Work out the finished part from the listing and answer in its coordinate system (mm). A direction names the side the tool comes from. Give positions to 0.01 mm unless a question says otherwise; leave off trailing zeros. Loops run counter-clockwise (first coordinate to the right, second up) from the corner with the lowest first, then second, coordinate; pieces in that order, holes last. Notation, with made-up numbers: (-4.75, -34) - (15.25, -34) arc R33 cw to (15.25, 5) - close; hole circle Ø10 at (71, -4.75). An arc over 180 degrees is marked (long way). Use CSV: the item, a comma, the result in double quotes.
from build123d import *

# Parameters (mm, degrees)
SKETCH1_R           = 4.25
SKETCH1_R_2         = 1.05
BOSS_EXTRUDE1_DEPTH = 23
BOSS_EXTRUDE3_DEPTH = 2
SKETCH4_W           = 21
SKETCH4_H           = 41
CUT_EXTRUDE1_DEPTH  = 50.288548817
BOSS_EXTRUDE4_START = 42
BOSS_EXTRUDE4_DEPTH = 42
CUT_EXTRUDE4_REACH  = 70.367


with BuildPart() as part:
    # Sketch1 → Boss-Extrude1 (new, symmetric)
    with BuildSketch(Plane.XY):
        with BuildLine():
            Line((-0.798015115, 9.968107738), (11.201984885, 9.968107738))
            ThreePointArc((11.201984885, 9.968107738), (19.90012903, 28.53283063), (7.687881875, 45))
            Line((7.687881875, 45), (3.464101615, 45))
            Line((3.464101615, 45), (0, 47))
            Line((0, 47), (10.5, 47))
            ThreePointArc((10.5, 47), (22.975048867, 25.465576737), (8.550692083, 5.18513885))
            ThreePointArc((8.550692083, 5.18513885), (-4.554689659, -8.902516617), (-0.798015115, 9.968107738))
        make_face()
        Circle(SKETCH1_R, mode=Mode.SUBTRACT)
        with Locations((0, 7)):
            Circle(SKETCH1_R_2, mode=Mode.SUBTRACT)
        with Locations((7, 0)):
            Circle(SKETCH1_R_2, mode=Mode.SUBTRACT)
        with Locations((0, -7)):
            Circle(SKETCH1_R_2, mode=Mode.SUBTRACT)
        with Locations((-7, 0)):
            Circle(SKETCH1_R_2, mode=Mode.SUBTRACT)
    extrude(amount=BOSS_EXTRUDE1_DEPTH, both=True)

    # Sketch3 → Boss-Extrude3 (add)
    with BuildSketch(Plane.XY.offset(23)):
        with BuildLine():
            Line((0, 47), (3.464101615, 45))
            Line((3.464101615, 45), (7.687881875, 45))
            ThreePointArc((7.687881875, 45), (19.90012903, 28.53283063), (11.201984885, 9.968107738))
            Line((11.201984885, 9.968107738), (0, 9.968107738))
            Line((0, 9.968107738), (0, 47))
        make_face()
    boss_extrude3 = extrude(amount=-BOSS_EXTRUDE3_DEPTH)

    # Mirror1: Boss-Extrude3 across plane
    add(boss_extrude3.mirror(Plane.XY))

    # Sketch4 → Cut-Extrude1 (cut, through all)
    with BuildSketch(Plane(origin=(0, 9.968107738, 0), x_dir=(1, 0, 0), z_dir=(0, 1, 0))):
        Rectangle(SKETCH4_W, SKETCH4_H)
    extrude(amount=-CUT_EXTRUDE1_DEPTH, mode=Mode.SUBTRACT)

    # Sketch6 → Boss-Extrude4 (add)
    with BuildSketch(Plane.XY.offset(-21).offset(BOSS_EXTRUDE4_START)):
        with BuildLine():
            Line((0, 22.833916422), (0, 19.973613057))
            ThreePointArc((0, 19.973613057), (8.195306737, 18.214888581), (14.947380695, 13.248434961))
            ThreePointArc((14.947380695, 13.248434961), (15.873509775, 14.369790734), (16.715701567, 15.555483287))
            ThreePointArc((16.715701567, 15.555483287), (9.115786688, 20.935380871), (0, 22.833916422))
        make_face()
    extrude(amount=-BOSS_EXTRUDE4_DEPTH)

    # Cut-Extrude4: up to this face of the body (flat: up to its plane)
    cut_extrude4_end = Plane(part.part.faces().sort_by_distance((6.103448613, 14.332073809, -21))[0])
    # Sketch7 → Cut-Extrude4 (cut, up to the picked face)
    with BuildSketch(Plane(origin=(0, 0, 21), x_dir=(-1, 0, 0), z_dir=(0, 0, -1)), mode=Mode.PRIVATE) as cut_extrude4_sk1:
        with BuildLine():
            Line((0, 19.973613057), (0, 9.968107738))
            ThreePointArc((0, 9.968107738), (-4.88859678, 8.68704745), (-8.520668778, 5.173139806))
            ThreePointArc((-8.520668778, 5.173139806), (-12.966457487, 7.54001363), (-16.790465857, 10.817831339))
            ThreePointArc((-16.790465857, 10.817831339), (-9.562270684, 17.535911665), (0, 19.973613057))
        make_face()
    cut_extrude4_tool1 = split(extrude(cut_extrude4_sk1.sketch, amount=CUT_EXTRUDE4_REACH, mode=Mode.PRIVATE), bisect_by=cut_extrude4_end, keep=Keep.BOTH, mode=Mode.PRIVATE)
    add(cut_extrude4_tool1.solids().sort_by(Axis((7.299259, 12.896939, 21), (0, 0, -1)))[0], mode=Mode.SUBTRACT)


solid = part.part
Item 1: A cutting plane is placed at A-A on y = 0. State how many separate pieces and enclosed holes the cut face has, and give its area (3 significant figures).
Determined:
separate pieces,"8"
enclosed holes,"0"
area,"36.5 mm²"
Item 2: Given P1, Ø7.5, axis at x = 0, y = 0, coming from the -Z side; P2, Ø4, axis at y = 12, z = -18, coming from the -X side; P3, Ø3, axis at y = 10.5, z = 12.5, coming from the -X side; P4, Ø0.9, axis at x = -0.5, z = -22, coming from the +Y side, each flat-ended and moving along its own axis, determine where each tip first touches the part or whether it passes through.
Determined:
P1,"passes through"
P2,"stops at x = 14.25"
P3,"stops at x = 15.97"
P4,"stops at y = 9.97"
Item 3: A cutting plane is placed at C-C on y = -7. Determine the outline of the cut face in (x, z), and give its area (3 significant figures).
Determined:
outline,"(-7.14, -23) - (-1.05, -23) - (-1.05, -20.5) - (-7.14, -20.5) - close; (-7.14, 20.5) - (-1.05, 20.5) - (-1.05, 23) - (-7.14, 23) - close; (1.05, -23) - (7.14, -23) - (7.14, -20.5) - (1.05, -20.5) - close; (1.05, 20.5) - (7.14, 20.5) - (7.14, 23) - (1.05, 23) - close"
area,"60.9 mm²"
Item 4: The mould has two halves that part along X. Classify faces 1 (the flat face through (7, 13, -21)), 2 (the cylindrical face through (19.192, 32.164, 0.294)), 3 (the cylindrical face through (4.83, 8.72, -20.75)), 4 (the cylindrical face through (-0.14, -5.96, 21.73)): pulls with the +X half, pulls with the -X half, needs draft (parallel to the pull), parting line crosses it, or undercut.
Determined:
face 1,"needs draft"
face 2,"undercut"
face 3,"pulls with the +X half"
face 4,"undercut"
Item 5: A cutting plane is placed at D-D on x = 12.5. Determine the outline of the cut face in (y, z), and give its area (3 significant figures).
Determined:
outline,"(7.23, -23) - (45.84, -23) - (45.84, 23) - (7.23, 23) - (7.23, 21) - (15.58, 21) - (15.58, -21) - (7.23, -21) - close; hole (19.11, -21) - (42.15, -21) - (42.15, 21) - (19.11, 21) - close"
area,"458 mm²"
Item 6: For faces 5 (the flat face through (6, 45, 0)), 6 (the cylindrical face through (5.95, 0.05, 21.73)), 7 (the flat face through (7, 13, 21)), determine the directions among +Z, -Z, +X, -X, +Y, -Y from which every point of the face is accessible in a straight line to the end or side of a thin tool.
Determined:
face 5,"-X"
face 6,"+Z, -Z"
face 7,"none"
Item 7: A cutting plane is placed at B-B on x = 7. Determine the outline of the cut face in (y, z).
Determined:
outline,"(-7.14, -23) - (-1.05, -23) - (-1.05, -20.5) - (-7.14, -20.5) - close; (-7.14, 20.5) - (-1.05, 20.5) - (-1.05, 23) - (-7.14, 23) - close; (1.05, -23) - (47, -23) - (47, 23) - (1.05, 23) - (1.05, 20.5) - (7.1, 20.5) - (7.1, 21) - (18.71, 21) - (18.71, -21) - (7.1, -21) - (7.1, -20.5) - (1.05, -20.5) - close; hole (21.73, -21) - (45, -21) - (45, 21) - (21.73, 21) - close"
Item 8: Find the intervals of material crossed by line 1 (X direction, y = 0, z = -21.05); line 2 (Z direction, x = 13, y = 8); line 3 (Z direction, x = -3.5, y = -7), in increasing order.
Determined:
line 1,"x = -10 to -8.05, -5.95 to -4.25, 4.25 to 5.95, 8.05 to 10"
line 2,"z = -23 to -21, 21 to 23"
line 3,"z = -23 to -20.5, 20.5 to 23"
